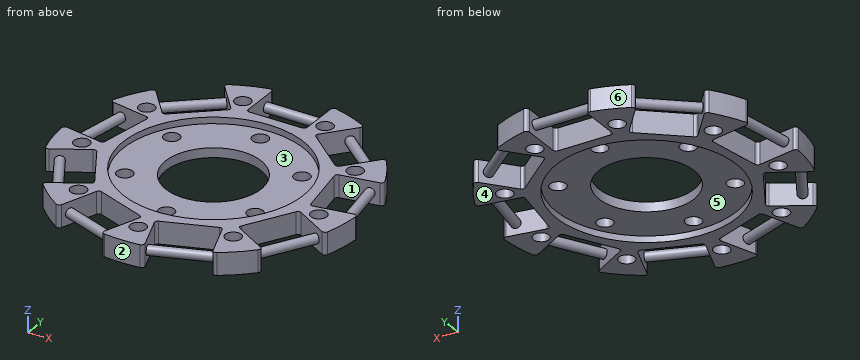
```python
from build123d import *

# Parameters (mm, degrees)
BOSS_EXTRUDE1_DEPTH      = 3.5
SKETCH3_R                = 2.5
CUT_EXTRUDE4_DEPTH       = 11
SKETCH7_R                = 28.35
CUT_EXTRUDE5_DEPTH       = 2
CUT_EXTRUDE6_START       = -2
SKETCH10_R               = 28.35
CUT_EXTRUDE6_DEPTH       = 2
SKETCH12_R               = 15
CUT_EXTRUDE7_DEPTH       = 66.909328951
SKETCH13_R               = 1.5
BOSS_EXTRUDE2_DEPTH      = 18.5
CIRPATTERN1_START        = -9.2
CIRPATTERN1_OUTLINE_R    = 1.5
CIRPATTERN1_DEPTH        = 18.5
CIRPATTERN1_2_OUTLINE_R  = 1.5
CIRPATTERN1_2_DEPTH      = 18.5
CIRPATTERN1_3_OUTLINE_R  = 1.5
CIRPATTERN1_3_DEPTH      = 18.5
CIRPATTERN1_START_2      = -9.3
CIRPATTERN1_4_OUTLINE_R  = 1.5
CIRPATTERN1_4_DEPTH      = 18.5
CIRPATTERN1_5_OUTLINE_R  = 1.5
CIRPATTERN1_5_DEPTH      = 18.5
CIRPATTERN1_6_OUTLINE_R  = 1.5
CIRPATTERN1_6_DEPTH      = 18.5
CIRPATTERN1_7_OUTLINE_R  = 1.5
CIRPATTERN1_7_DEPTH      = 18.5
CIRPATTERN1_8_OUTLINE_R  = 1.5
CIRPATTERN1_8_DEPTH      = 18.5
SKETCH_1_R               = 2.5
CUT_EXTRUDE_1_DEPTH      = 66.909328951
PATTERN_CIRCULAR_1_COUNT = 6


# Read off the part's stored shape, not the designer's step: CirPattern1
with BuildPart() as part:
    # Sketch1 → Boss-Extrude1 (new, symmetric)
    with BuildSketch(Plane.XY):
        with BuildLine():
            Line((8.3, 31.537634409), (-8.3, 31.537634409))
            ThreePointArc((-8.3, 31.537634409), (-9.007106781, 31.830527627), (-9.3, 32.537634409))
            Line((-9.3, 32.537634409), (-9.3, 44.322482838))
            ThreePointArc((-9.3, 44.322482838), (-9.67804984, 45.105539668), (-10.526355997, 45.296527479))
            ThreePointArc((-10.526355997, 45.296527479), (-15.905148665, 43.699036811), (-21.052390107, 41.465364378))
            ThreePointArc((-21.052390107, 41.465364378), (-21.579465726, 40.773778539), (-21.365729478, 39.930916453))
            Line((-21.365729478, 39.930916453), (-13.790574925, 30.903198801))
            ThreePointArc((-13.790574925, 30.903198801), (-13.56042467, 30.173255449), (-13.913831759, 29.494366748))
            Line((-13.913831759, 29.494366748), (-26.630169515, 18.824092427))
            ThreePointArc((-26.630169515, 18.824092427), (-27.360112867, 18.593942172), (-28.039001567, 18.947349261))
            Line((-28.039001567, 18.947349261), (-35.61415612, 27.975066913))
            ThreePointArc((-35.61415612, 27.975066913), (-36.407098327, 28.331917493), (-37.179703143, 27.932941958))
            ThreePointArc((-37.179703143, 27.932941958), (-40.273250169, 23.251771826), (-42.780488909, 18.232096448))
            ThreePointArc((-42.780488909, 18.232096448), (-42.73970945, 17.363513283), (-42.034196679, 16.855230478))
            Line((-42.034196679, 16.855230478), (-30.428386578, 14.808813024))
            ThreePointArc((-30.428386578, 14.808813024), (-29.782882711, 14.397581707), (-29.617227003, 13.650357093))
            Line((-29.617227003, 13.650357093), (-32.499786752, -2.697451607))
            ThreePointArc((-32.499786752, -2.697451607), (-32.911018069, -3.342955474), (-33.658242683, -3.508611182))
            Line((-33.658242683, -3.508611182), (-45.264052784, -1.462193729))
            ThreePointArc((-45.264052784, -1.462193729), (-46.100860887, -1.698523751), (-46.436253982, -2.500777546))
            ThreePointArc((-46.436253982, -2.500777546), (-45.797050331, -8.07525561), (-44.491121499, -13.532172037))
            ThreePointArc((-44.491121499, -13.532172037), (-43.901568124, -14.171332813), (-43.034396096, -14.107205164))
            Line((-43.034396096, -14.107205164), (-32.828417977, -8.214780949))
            ThreePointArc((-32.828417977, -8.214780949), (-32.069598932, -8.114880527), (-31.462392573, -8.580806353))
            Line((-31.462392573, -8.580806353), (-23.162392573, -22.956828056))
            ThreePointArc((-23.162392573, -22.956828056), (-23.062492151, -23.715647101), (-23.528417977, -24.322853459))
            Line((-23.528417977, -24.322853459), (-33.734396096, -30.215277674))
            ThreePointArc((-33.734396096, -30.215277674), (-34.223518284, -30.934206854), (-33.964765501, -31.764355442))
            ThreePointArc((-33.964765501, -31.764355442), (-29.891901666, -35.6237812), (-25.383863875, -38.964586832))
            ThreePointArc((-25.383863875, -38.964586832), (-24.52139516, -39.075254789), (-23.898323306, -38.468722725))
            Line((-23.898323306, -38.468722725), (-19.867667757, -27.394587619))
            ThreePointArc((-19.867667757, -27.394587619), (-19.350593398, -26.830299975), (-18.585954993, -26.796915141))
            Line((-18.585954993, -26.796915141), (-2.987057488, -32.47444952))
            ThreePointArc((-2.987057488, -32.47444952), (-2.422769844, -32.991523879), (-2.389385011, -33.756162285))
            Line((-2.389385011, -33.756162285), (-6.420040559, -44.830297391))
            ThreePointArc((-6.420040559, -44.830297391), (-6.332611124, -45.695430776), (-5.600785766, -46.165038406))
            ThreePointArc((-5.600785766, -46.165038406), (0, -46.503543652), (5.600785766, -46.165038406))
            ThreePointArc((5.600785766, -46.165038406), (6.332611124, -45.695430776), (6.420040559, -44.830297391))
            Line((6.420040559, -44.830297391), (2.389385011, -33.756162285))
            ThreePointArc((2.389385011, -33.756162285), (2.422769844, -32.991523879), (2.987057488, -32.47444952))
            Line((2.987057488, -32.47444952), (18.585954993, -26.796915141))
            ThreePointArc((18.585954993, -26.796915141), (19.350593398, -26.830299975), (19.867667757, -27.394587619))
            Line((19.867667757, -27.394587619), (23.898323306, -38.468722725))
            ThreePointArc((23.898323306, -38.468722725), (24.52139516, -39.075254789), (25.383863875, -38.964586832))
            ThreePointArc((25.383863875, -38.964586832), (29.891901666, -35.6237812), (33.964765501, -31.764355442))
            ThreePointArc((33.964765501, -31.764355442), (34.223518284, -30.934206854), (33.734396096, -30.215277674))
            Line((33.734396096, -30.215277674), (23.528417977, -24.322853459))
            ThreePointArc((23.528417977, -24.322853459), (23.062492151, -23.715647101), (23.162392573, -22.956828056))
            Line((23.162392573, -22.956828056), (31.462392573, -8.580806353))
            ThreePointArc((31.462392573, -8.580806353), (32.069598932, -8.114880527), (32.828417977, -8.214780949))
            Line((32.828417977, -8.214780949), (43.034396096, -14.107205164))
            ThreePointArc((43.034396096, -14.107205164), (43.901568124, -14.171332813), (44.491121499, -13.532172037))
            ThreePointArc((44.491121499, -13.532172037), (45.797050331, -8.07525561), (46.436253982, -2.500777546))
            ThreePointArc((46.436253982, -2.500777546), (46.100860887, -1.698523751), (45.264052784, -1.462193729))
            Line((45.264052784, -1.462193729), (33.658242683, -3.508611182))
            ThreePointArc((33.658242683, -3.508611182), (32.911018069, -3.342955474), (32.499786752, -2.697451607))
            Line((32.499786752, -2.697451607), (29.617227003, 13.650357093))
            ThreePointArc((29.617227003, 13.650357093), (29.782882711, 14.397581707), (30.428386578, 14.808813024))
            Line((30.428386578, 14.808813024), (42.034196679, 16.855230478))
            ThreePointArc((42.034196679, 16.855230478), (42.73970945, 17.363513283), (42.780488909, 18.232096448))
            ThreePointArc((42.780488909, 18.232096448), (40.273250169, 23.251771826), (37.179703143, 27.932941958))
            ThreePointArc((37.179703143, 27.932941958), (36.407098327, 28.331917493), (35.61415612, 27.975066913))
            Line((35.61415612, 27.975066913), (28.039001567, 18.947349261))
            ThreePointArc((28.039001567, 18.947349261), (27.360112867, 18.593942172), (26.630169515, 18.824092427))
            Line((26.630169515, 18.824092427), (13.913831759, 29.494366748))
            ThreePointArc((13.913831759, 29.494366748), (13.56042467, 30.173255449), (13.790574925, 30.903198801))
            Line((13.790574925, 30.903198801), (21.365729478, 39.930916453))
            ThreePointArc((21.365729478, 39.930916453), (21.579465726, 40.773778539), (21.052390107, 41.465364378))
            ThreePointArc((21.052390107, 41.465364378), (15.905148665, 43.699036811), (10.526355997, 45.296527479))
            ThreePointArc((10.526355997, 45.296527479), (9.67804984, 45.105539668), (9.3, 44.322482838))
            Line((9.3, 44.322482838), (9.3, 32.537634409))
            ThreePointArc((9.3, 32.537634409), (9.007106781, 31.830527627), (8.3, 31.537634409))
        make_face()
    extrude(amount=BOSS_EXTRUDE1_DEPTH, both=True)

    # Sketch3 → Cut-Extrude4 (cut)
    with BuildSketch(Plane.XY.offset(3.5)):
        with Locations((12.996765446, 35.70831959)):
            Circle(SKETCH3_R)
        with Locations((-12.996765446, 35.70831959)):
            Circle(SKETCH3_R)
        with Locations((32.908965344, 19)):
            Circle(SKETCH3_R)
        with Locations((37.422694614, -6.598630751)):
            Circle(SKETCH3_R)
        with Locations((24.425929168, -29.109688839)):
            Circle(SKETCH3_R)
        with Locations((0, -38)):
            Circle(SKETCH3_R)
        with Locations((-24.425929168, -29.109688839)):
            Circle(SKETCH3_R)
        with Locations((-37.422694614, -6.598630751)):
            Circle(SKETCH3_R)
        with Locations((-32.908965344, 19)):
            Circle(SKETCH3_R)
    extrude(amount=-CUT_EXTRUDE4_DEPTH, mode=Mode.SUBTRACT)

    # Sketch7 → Cut-Extrude5 (cut)
    with BuildSketch(Plane.XY.offset(3.5)):
        Circle(SKETCH7_R)
    extrude(amount=-CUT_EXTRUDE5_DEPTH, mode=Mode.SUBTRACT)

    # Sketch10 → Cut-Extrude6 (cut)
    with BuildSketch(Plane(origin=(0, 0, -3.5), x_dir=(-1, 0, 0), z_dir=(0, 0, -1)).offset(CUT_EXTRUDE6_START)):
        with Locations(Location((0, 0, 0), (0, 0, 180))):
            Circle(SKETCH10_R)
    extrude(amount=CUT_EXTRUDE6_DEPTH, mode=Mode.SUBTRACT)

    # Sketch12 → Cut-Extrude7 (cut, through all)
    with BuildSketch(Plane(origin=(0, 0, -1.5), x_dir=(-1, 0, 0), z_dir=(0, 0, -1))):
        Circle(SKETCH12_R)
    extrude(amount=-CUT_EXTRUDE7_DEPTH, mode=Mode.SUBTRACT)

    # Sketch13 → Boss-Extrude2 (add)
    with BuildSketch(Plane(origin=(7.124213321, -5.97792477, 0), x_dir=(0, 0, 1), z_dir=(-0.7660444431189782, 0.6427876096865393, 0))):
        with Locations(Location((0, 41.5, 0), (0, 0, 90))):
            Circle(SKETCH13_R)
    extrude(amount=BOSS_EXTRUDE2_DEPTH)

    # CirPattern1 outline → CirPattern1 (add)
    with BuildSketch(Plane.YZ.offset(CIRPATTERN1_START)):
        with Locations((41.5, 0)):
            Circle(CIRPATTERN1_OUTLINE_R)
    extrude(amount=CIRPATTERN1_DEPTH)

    # CirPattern1 2 outline → CirPattern1 2 (add)
    with BuildSketch(Plane(origin=(0, 0, 0), x_dir=(0.6427876096865098, -0.7660444431190029, 0), z_dir=(0.7660444431190028, 0.6427876096865099, 0)).offset(CIRPATTERN1_START)):
        with Locations((-41.5, 0)):
            Circle(CIRPATTERN1_2_OUTLINE_R)
    extrude(amount=CIRPATTERN1_2_DEPTH)

    # CirPattern1 3 outline → CirPattern1 3 (add)
    with BuildSketch(Plane(origin=(0, 0, 0), x_dir=(0.9848077530121979, -0.17364817766698804, 0), z_dir=(0.173648177666988, 0.984807753012198, 0)).offset(CIRPATTERN1_START)):
        with Locations((-41.5, 0)):
            Circle(CIRPATTERN1_3_OUTLINE_R)
    extrude(amount=CIRPATTERN1_3_DEPTH)

    # CirPattern1 4 outline → CirPattern1 4 (add)
    with BuildSketch(Plane(origin=(0, 0, 0), x_dir=(0.8660254037844768, 0.49999999999993383, 0), z_dir=(0.4999999999999339, -0.8660254037844768, 0)).offset(CIRPATTERN1_START_2)):
        with Locations((-41.5, 0)):
            Circle(CIRPATTERN1_4_OUTLINE_R)
    extrude(amount=CIRPATTERN1_4_DEPTH)

    # CirPattern1 5 outline → CirPattern1 5 (add)
    with BuildSketch(Plane(origin=(0, 0, 0), x_dir=(0.34202014332575803, 0.9396926207858759, 0), z_dir=(0.939692620785876, -0.342020143325758, 0)).offset(CIRPATTERN1_START_2)):
        with Locations((-41.5, 0)):
            Circle(CIRPATTERN1_5_OUTLINE_R)
    extrude(amount=CIRPATTERN1_5_DEPTH)

    # CirPattern1 6 outline → CirPattern1 6 (add)
    with BuildSketch(Plane(origin=(0, 0, 0), x_dir=(-0.34202014332555913, 0.9396926207859483, 0), z_dir=(0.9396926207859483, 0.34202014332555913, 0)).offset(CIRPATTERN1_START_2)):
        with Locations((-41.5, 0)):
            Circle(CIRPATTERN1_6_OUTLINE_R)
    extrude(amount=CIRPATTERN1_6_DEPTH)

    # CirPattern1 7 outline → CirPattern1 7 (add)
    with BuildSketch(Plane(origin=(0, 0, 0), x_dir=(0.8660254037843728, -0.500000000000114, 0), z_dir=(0.500000000000114, 0.8660254037843729, 0)).offset(CIRPATTERN1_START_2)):
        with Locations((41.5, 0)):
            Circle(CIRPATTERN1_7_OUTLINE_R)
    extrude(amount=CIRPATTERN1_7_DEPTH)

    # CirPattern1 8 outline → CirPattern1 8 (add)
    with BuildSketch(Plane(origin=(0, 0, 0), x_dir=(0.9848077530122347, 0.17364817766677898, 0), z_dir=(0.17364817766677898, -0.9848077530122348, 0)).offset(CIRPATTERN1_START)):
        with Locations((41.5, 0)):
            Circle(CIRPATTERN1_8_OUTLINE_R)
    extrude(amount=CIRPATTERN1_8_DEPTH)

    # 草圖1 → 除料-伸長1 (cut, through all)
    with BuildSketch(Plane.XY.offset(1.5)):
        with Locations((0, 23.75)):
            Circle(SKETCH_1_R)
    cut_extrude_1 = extrude(amount=-CUT_EXTRUDE_1_DEPTH, mode=Mode.SUBTRACT)

    # 環狀複製排列1: 除料-伸長1 ×6 about axis
    pattern_circular_1_axis = Axis((0, 0, 0), (0, 0, 1))
    for i in range(1, PATTERN_CIRCULAR_1_COUNT):
        add(cut_extrude_1.rotate(pattern_circular_1_axis, i * 360 / PATTERN_CIRCULAR_1_COUNT), mode=Mode.SUBTRACT)


solid = part.part
```
Input: part model. Units: mm. Frame: model coordinates. Face numbers are marked on the shaded views. A direction names the side the tool comes from. Coordinates: 2 decimals unless noted, no trailing zeros. Return JSON: item names as keys, results as strings.
Q1. First-contact query: pin 1 (4.5 mm diameter, centred on x = -20.57, y = 11.88, fed in from +Z); pin 2 (4 mm diameter, centred on y = 18.5, z = 1.5, fed in from +X); pin 3 (3.5 mm diameter, centred on y = 38, z = 1.5, fed in from -X); pin 4 (1.5 mm diameter, centred on y = 42, z = 0.5, fed in from -X). Flat tips, straight axial feed; report the tip coordinate or a pass-through.
The answers:
{"pin 1": "passes through", "pin 2": "stops at x = 42.86", "pin 3": "stops at x = -23.2", "pin 4": "stops at x = -21.34"}
Q2. Ray query, probe 1 along X at (y, z) = (-5, 0); probe 2 along X at (y, z) = (-25, -0.5); probe 3 along Y at (x, z) = (-33, 1.75). Return the intervals inside material, ascending.
The answers:
{"probe 1": "x = -46.23 to -39.34, -35.5 to -14.14, 14.14 to 35.5, 39.34 to 46.23", "probe 2": "x = -35.12 to -31.85, -24.7 to -2.17, 2.17 to 24.7, 31.85 to 35.12", "probe 3": "y = -32.77 to -29.79, -8.31 to -3.4, 15.26 to 16.5, 21.5 to 24.86"}
Q3. Cut plane A-A (x = 0). State how many separate pieces and enclosed holes the cut face has, then the cut area to 3 significant figures.
The answers:
{"separate pieces": "6", "enclosed holes": "0", "area": "172 mm2"}
Q4. Draft query along Y for the marked faces 4, 5 and 6. Return one class per face: +Y half, -Y half, draft (parallel to the pull), parting line (faces both ways), or undercut.
The answers:
{"face 4": "draft", "face 5": "undercut", "face 6": "+Y half"}
Q5. Access query for the marked faces 1, 2 and 3. Directions: +Z, -Z, +X, -X, +Y, -Y. A direction counts if a zero-diameter tool reaches every point of the face in a straight line with its end or side. Return the directions, or none.
The answers:
{"face 1": "+Z, -Z", "face 2": "+Z, -Z, -Y", "face 3": "+Z"}
